CAD build for the part. Positions are in the model's coordinates, mm. Face numbers are marked on the shaded views. Coordinates: 2 decimals unless noted, no trailing zeros. Loops run counter-clockwise (first coordinate to the right, second up) from the corner with the lowest first, then second, coordinate; pieces in that order, holes last. Notation, with made-up numbers: (-9.75, 39.25) -> (-5.75, 39.25) arc R30 cw to (-5.75, 73.25) -> close; hole circle Ø5 at (-28, -22.75). An arc over 180 degrees is marked (long way). Return JSON: item names as keys, results as strings. Group by question number.
(1) Saw through at B-B on z = 3.5. Write the cut outline in (x, y).
(2) Saw through at C-C on y = -4. Write the cut outline in (x, z).
(3) Probe L1, parallel to Y at x = 19, z = 2; L2, parallel to Z at x = 12.5, y = 0; L3, parallel to Y at x = 8, z = 0.5. List the from-to ranges inside material, lowest first.
(4) Mould opens along Z. For the marked faces 1, 2 and 3 say: pulls with the +Z half, pulls with the -Z half, needs draft (parallel to the pull), parting line crosses it, or undercut.
(5) Saw through at A-A on x = 4. Write the cut outline in (y, z), then the cut area to 3 significant figures.
(6) Flat gauge pins, fed straight in: pin 1 Ø5 at (x, z) = (11, 2) entering from -Y; pin 2 Ø3 at (x, z) = (18, 3.5) entering from -Y; pin 3 Ø3 at (x, y) = (25, -1) entering from -Z; pin 4 Ø4 at (x, y) = (4.5, -0.5) entering from -Z. Where does each tip first touch, or does it go through?
```python
from build123d import *

# Parameters (mm, degrees)
FILLET_1_R  = 0.2
HEX_2_DEPTH = 1.56


with BuildPart() as part:
    # Эскиз1 → Body (revolve)
    with BuildSketch(Plane.XY):
        with BuildLine():
            Line((0, 2.375), (0, 0))
            Line((0, 0), (37.75, 0))
            Line((37.75, 0), (37.75, 2.055))
            Line((37.75, 2.055), (37.305, 2.5))
            Line((37.305, 2.5), (2.75, 2.5))
            Line((2.75, 2.5), (2.75, 4.75))
            Line((2.75, 4.75), (2.370164642, 4.75))
            ThreePointArc((2.370164642, 4.75), (0.992749859, 3.754440885), (0, 2.375))
        make_face()
    revolve(axis=Axis((-3.643489966, 0, 0), (-1, 0, 0)))

    # Скругление1
    fillet_1_edges = [part.edges().sort_by_distance(p)[0] for p in [
        (2.75, -2.5, 0),
    ]]
    fillet(fillet_1_edges, radius=FILLET_1_R)

    # Эскиз2 → Вырез-Повернуть1 (revolve, cut)
    with BuildSketch(Plane.XY):
        Polygon((0, 0), (0, 1.5), (1.56, 1.5), (2.426025404, 0), align=None)
    revolve(axis=Axis((2.426025404, 0, 0), (-1, 0, 0)), mode=Mode.SUBTRACT)

    # Эскиз3 → Hex 2 (cut)
    with BuildSketch(Plane.ZY):
        Polygon((-1.5, -0.866025404), (0, -1.732050808), (1.5, -0.866025404), (1.5, 0.866025404), (0, 1.732050808), (-1.5, 0.866025404), align=None)
    extrude(amount=-HEX_2_DEPTH, mode=Mode.SUBTRACT)


solid = part.part
```
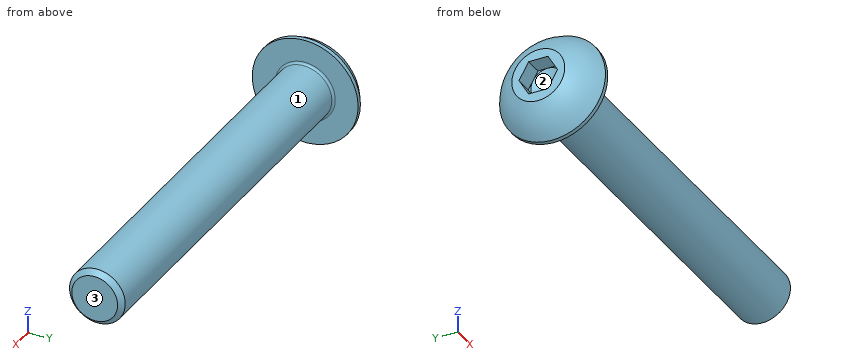
Geometry results:
{
 "1": {"outline": "(2.37, -3.21) -> (2.75, -3.21) -> (2.75, 3.21) -> (2.37, 3.21) arc R4 ccw to start"},
 "2": {"outline": "(2.37, -2.56) -> (2.75, -2.56) -> (2.75, 2.56) -> (2.37, 2.56) arc R3.5 ccw to start"},
 "3": {"L1": "-1.5 to 1.5", "L2": "-2.5 to 2.5", "L3": "-2.45 to 2.45"},
 "4": {"face 1": "parting line crosses it", "face 2": "undercut", "face 3": "needs draft"},
 "5": {"outline": "circle Ø5 at (0, 0)", "area": "19.6 mm²"},
 "6": {"pin 1": "y = -2.5", "pin 2": "y = -1.5", "pin 3": "z = -2.5", "pin 4": "z = -4.75"}
}
